Answer from the drawing. Dimensions are ordinates in mm from the lowest x, y and z of the part. Coordinates: 2 decimals unless noted, no trailing zeros. Loops run counter-clockwise (first coordinate to the right, second up) from the corner with the lowest first, then second, coordinate; pieces in that order, holes last.
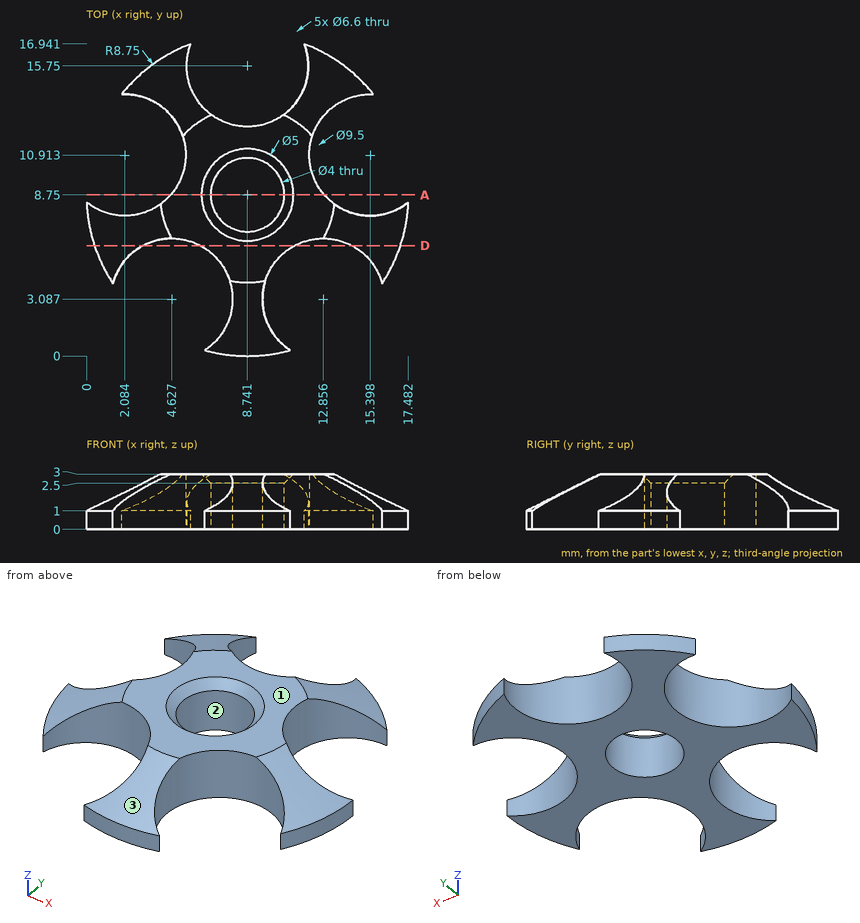
Item 1: Given pin 1 (5.5 mm diameter, centred on x = 8.74, y = 15.75, fed in from -Z); pin 2 (1 mm diameter, centred on y = 7, z = 1, fed in from +X); pin 3 (5 mm diameter, centred on x = 12.5, y = 13.5, fed in from +Z), each flat-ended and moving along its own axis, determine where each tip first touches the part or whether it passes through.
Numbers:
pin 1: passes through
pin 2: stops at x = 17.4
pin 3: stops at z = 3
Item 2: Find the intervals of material crossed by line 1 along Y through (x, z) = (7.5, 0.8) (1 decimal); line 2 along X through (y, z) = (11, 2.7); line 3 along X through (y, z) = (13, 0.75) (1 decimal), in increasing order.
Numbers:
line 1: y = 0.1 to 1.5, 4.7 to 7.2, 10.3 to 12.7
line 2: x = 5.38 to 12.1
line 3: x = 4.6 to 6.9, 10.6 to 12.8
Item 3: A cutting plane is placed at D-D on y = 6. Give the number of separate pieces and of enclosed holes in the cut face.
Numbers:
separate pieces: 3
enclosed holes: 0
Item 4: A cutting plane is placed at A-A on y = 8.75. Determine the outline of the cut face in (x, z) (1 decimal).
Numbers:
outline: (4.6, 0) - (6.7, 0) - (6.7, 2.5) - (6.2, 3) - (4.6, 3) - close; (10.7, 0) - (12.9, 0) - (12.9, 3) - (11.2, 3) - (10.7, 2.5) - close
Item 5: Determine the mould class of the marked faces 1, 2 and 3 for opening direction Y: released by +Y, released by -Y, zero draft, split by the parting line, or undercut.
Numbers:
face 1: zero draft
face 2: undercut
face 3: released by -Y
